Source: CAD feature listing. Evaluate the final solid. Frame: model axes, mm. A direction names the side the tool comes from. Give positions to 0.01 mm unless a question says otherwise; leave off trailing zeros. Write each loop counter-clockwise with the first axis right and the second up, starting at its lowest first coordinate (ties: lowest second). Pieces come first, ordered by that corner, then holes. Notation, with made-up numbers: M 68,87.25 L 78,87.25 A33 ccw 78,124.25 Z; hole C 54.25,12 d10. An arc over 180 degrees is marked long. Return JSON: item names as keys, results as strings.
```python
from build123d import *

# Parameters (mm, degrees)
SKETCH1_W          = 10.0076
SKETCH1_H          = 13.0048
EXTRUDE1_DEPTH     = 10.0076
SKETCH2_R          = 4.445
EXTRUDE2_DEPTH     = 9.4996
FILLET1_R          = 0.762
SKETCH3_R          = 1.64973
CUT_EXTRUDE1_DEPTH = 9.4996
CUT_EXTRUDE2_DEPTH = 0.6096
SKETCH5_W          = 1.082217623
SKETCH5_H          = 7.941923042
CUT_EXTRUDE3_DEPTH = 11.0076
SKETCH6_W          = 7.62
SKETCH6_H          = 1.4986
CUT_EXTRUDE4_DEPTH = 11.0076
SKETCH7_R          = 2.588003294
CUT_EXTRUDE5_DEPTH = 1.27
SKETCH8_W          = 3.9878
SKETCH8_H          = 0.5588
CUT_EXTRUDE6_DEPTH = 11.0076
SKETCH10_W         = 8.302680101
SKETCH10_H         = 1.4986
CUT_EXTRUDE8_DEPTH = 11.0076
SKETCH11_W         = 0.763867388
SKETCH11_H         = 0.721519404
CUT_EXTRUDE9_DEPTH = 11.0076
SKETCH12_W         = 2.0066
SKETCH12_H         = 0.381
FILLET2_R          = 0.9906
EXTRUDE3_DEPTH     = 0.254


with BuildPart() as part:
    # Sketch1 → Extrude1 (new body)
    with BuildSketch(Plane.XY):
        with Locations((0, 6.5024)):
            Rectangle(SKETCH1_W, SKETCH1_H)
    extrude(amount=-EXTRUDE1_DEPTH)

    # Sketch2 → Extrude2 (add)
    with BuildSketch(Plane.XY):
        with Locations((0, 8.001)):
            Circle(SKETCH2_R)
    extrude(amount=EXTRUDE2_DEPTH)

    # Fillet1
    fillet1_edges = [part.edges().sort_by_distance(p)[0] for p in [
        (-4.445, 8.001, 9.4996),
    ]]
    fillet(fillet1_edges, radius=FILLET1_R)

    # Sketch3 → Cut-Extrude1 (cut)
    with BuildSketch(Plane.XY.offset(9.4996)):
        with Locations((0, 8.001)):
            Circle(SKETCH3_R)
    extrude(amount=-CUT_EXTRUDE1_DEPTH, mode=Mode.SUBTRACT)

    # Sketch4 → Cut-Extrude2 (cut)
    with BuildSketch(Plane(origin=(5.0038, 0, 0), x_dir=(0, 0, -1), z_dir=(1, 0, 0))):
        Polygon((0, 8.9535), (7.063951239, 8.9535), (7.063951239, 7.0485), (0.484947525, 7.0485), (0.484947525, 3.872808147), (0, 3.872808147), align=None)
    cut_extrude2 = extrude(amount=-CUT_EXTRUDE2_DEPTH, mode=Mode.SUBTRACT)

    # Sketch5 → Cut-Extrude3 (cut, through all)
    with BuildSketch(Plane(origin=(5.0038, 0, 0), x_dir=(0, 0, -1), z_dir=(1, 0, 0))):
        with Locations((9.466491189, 8.113930335)):
            Rectangle(SKETCH5_W, SKETCH5_H)
    extrude(amount=-CUT_EXTRUDE3_DEPTH, mode=Mode.SUBTRACT)

    # Sketch6 → Cut-Extrude4 (cut, through all)
    with BuildSketch(Plane.XY):
        with Locations((0, 0.7493)):
            Rectangle(SKETCH6_W, SKETCH6_H)
    extrude(amount=-CUT_EXTRUDE4_DEPTH, mode=Mode.SUBTRACT)

    # Sketch7 → Cut-Extrude5 (cut)
    with BuildSketch(Plane.XY.offset(9.4996)):
        with Locations((0, 8.001)):
            Circle(SKETCH7_R)
    extrude(amount=-CUT_EXTRUDE5_DEPTH, mode=Mode.SUBTRACT)

    # Sketch8 → Cut-Extrude6 (cut, through all)
    with BuildSketch(Plane.XY):
        with Locations((0, 12.7254)):
            Rectangle(SKETCH8_W, SKETCH8_H)
    extrude(amount=-CUT_EXTRUDE6_DEPTH, mode=Mode.SUBTRACT)

    # Mirror1: Cut-Extrude2 across plane
    add(cut_extrude2.mirror(Plane(origin=(0, 0, 0), x_dir=(0, 0, 1), z_dir=(1, 0, 0))), mode=Mode.SUBTRACT)

    # Sketch10 → Cut-Extrude8 (cut, through all)
    with BuildSketch(Plane(origin=(5.0038, 0, 0), x_dir=(0, 0, -1), z_dir=(1, 0, 0))):
        with Locations((5.85625995, 0.7493)):
            Rectangle(SKETCH10_W, SKETCH10_H)
    extrude(amount=-CUT_EXTRUDE8_DEPTH, mode=Mode.SUBTRACT)

    # Sketch11 → Cut-Extrude9 (cut, through all)
    with BuildSketch(Plane(origin=(5.0038, 0, 0), x_dir=(0, 0, -1), z_dir=(1, 0, 0))):
        with Locations((9.625666306, 3.782209112)):
            Rectangle(SKETCH11_W, SKETCH11_H)
    extrude(amount=-CUT_EXTRUDE9_DEPTH, mode=Mode.SUBTRACT)

    # Sweep1: sweep along a path in Sketch13
    with BuildLine(Plane(origin=(0, 0, 0), x_dir=(0, 0, -1), z_dir=(1, 0, 0))) as sweep1_path:
        Line((3.9878, 1.4986), (3.9878, 0.118233573))
        ThreePointArc((3.9878, 0.118233573), (3.963359224, -0.233279995), (3.890507253, -0.578028788))
        ThreePointArc((3.890507253, -0.578028788), (3.561195264, -1.630409905), (3.70889827, -2.723175307))
        Line((3.70889827, -2.723175307), (3.9878, -3.4798))
        Line((3.9878, -3.4798), (3.9878, -3.9878))
    # Sketch12 → Sweep1 (sweep)
    with BuildSketch(Plane.XZ.offset(-1.4986)):
        with Locations((0, -3.9878)):
            Rectangle(SKETCH12_W, SKETCH12_H)
    sweep(path=sweep1_path.line, transition=Transition.RIGHT)

    # Fillet2
    fillet2_edges = [part.edges().sort_by_distance(p)[0] for p in [
        (1.0033, -3.9878, -3.9878),
        (-1.0033, -3.9878, -3.9878),
    ]]
    fillet(fillet2_edges, radius=FILLET2_R)

    # Sketch14 → Extrude3 (add, symmetric)
    with BuildSketch(Plane(origin=(0, 0, 0), x_dir=(0, 0, -1), z_dir=(1, 0, 0))):
        with BuildLine():
            Line((10.007599936, 0), (9.055129464, 0))
            Line((9.055129464, 0), (9.055129464, -1.459458075))
            Line((9.055129464, -1.459458075), (10.007599936, -1.950513398))
            Line((10.007599936, -1.950513398), (9.466255271, -3.000527083))
            ThreePointArc((9.466255271, -3.000527083), (8.363488428, -3.473928976), (7.628868664, -2.52496224))
            Line((7.628868664, -2.52496224), (7.628868664, 1.4986))
            Line((7.628868664, 1.4986), (10.007599936, 1.4986))
            Line((10.007599936, 1.4986), (10.007599936, 0))
        make_face()
    extrude(amount=EXTRUDE3_DEPTH, both=True)


solid = part.part
```
1) Contact query for flat-ended pins moving along their axis: pin 1 Ø2 at (x, y) = (0.5, 6.5) entering from -Z; pin 2 Ø0.6 at (x, y) = (0, -4) entering from -Z; pin 3 Ø0.6 at (x, z) = (-4.5, -0.5) entering from -Y. Output: stop coordinate, or through.
Numbers:
{"pin 1": "stops at z = -8.93", "pin 2": "stops at z = -4.18", "pin 3": "stops at y = 0"}
2) Draft query along X for faces 1 (the face through (-0.561, 5.475, 8.873)), 2 (the face through (1.003, -0.8, -3.8)), 3 (the face through (-1.003, -0.8, -3.8)). Return one class per face: released by +X, released by -X, zero draft, split by the parting line, or undercut.
Numbers:
{"face 1": "undercut", "face 2": "released by +X", "face 3": "released by -X"}
3) Cut plane B-B, the plane z = -0.25. Return the cut outline in (x, y).
Numbers:
{"outline": "M -5,0 L -3.81,0 L -3.81,1.5 L 3.81,1.5 L 3.81,0 L 5,0 L 5,3.87 L 4.39,3.87 L 4.39,8.95 L 5,8.95 L 5,13 L 1.99,13 L 1.99,12.45 L -1.99,12.45 L -1.99,13 L -5,13 L -5,8.95 L -4.39,8.95 L -4.39,3.87 L -5,3.87 Z"}
4) Cut plane A-A, the plane z = -5.5. Return the cut outline in (x, y), then the cut area to 3 significant figures.
Numbers:
{"outline": "M -5,1.5 L 5,1.5 L 5,7.05 L 4.39,7.05 L 4.39,8.95 L 5,8.95 L 5,13 L 1.99,13 L 1.99,12.45 L -1.99,12.45 L -1.99,13 L -5,13 L -5,8.95 L -4.39,8.95 L -4.39,7.05 L -5,7.05 Z", "area": "111 mm²"}
5) Set-up query: faces 4 (the face through (2, 8, 8.23)), 5 (the face through (5.004, 6, -5)), 6 (the face through (4, 12, 0)), 7 (the face through (0, 1, -4.178)), 8 (the face through (-3.81, 1, -1)). Return all of +Z, -Z, +X, -X, +Y, -Y with unobstructed straight access to the full face (end or side cutting, diameter ignored); none if empty.
Numbers:
{"face 4": "+Z", "face 5": "+Z, -Z, +X, +Y, -Y", "face 6": "+Z, +X, +Y", "face 7": "+X, -X, -Y", "face 8": "+Z, -Z, -Y"}
6) Line query: line 1 (Y direction, x = 0, z = 6.5); line 2 (Y direction, x = 4.5, z = -7); line 3 (Z direction, x = 1, y = 10). Output: solid intervals per line, ascending. Write a range as [from, to].
Numbers:
{"line 1": "y = [3.56, 6.35], [9.65, 12.45]", "line 2": "y = [1.5, 7.05], [8.95, 13]", "line 3": "z = [-8.93, 8.23]"}
